Could you check a few things on this model? Use its own coordinates, in mm. A direction names the side the tool comes from. Coordinates: 2 decimals unless noted, no trailing zeros. Order: outer loops, then holes, each group sorted by start corner. A loop starts at its lowest first (then second) coordinate and runs counter-clockwise, first axis right, second up. Notation, with made-up numbers: (31.5, -22) - (62.5, -22) arc R20 cw to (62.5, 1) - close; hole circle Ø3 at (-32, -33). An arc over 180 degrees is marked (long way). Answer as CSV lines item,"result". Start each with the question number.
1. I want a section at B-B, the plane x = 13.25. List the corners of the cut face in (y, z) for me (3 decimals), and give its area (3 significant figures).
2. I want a section at A-A, the plane z = 0. List the corners of the cut face in (x, y) for me (3 decimals), and give its area (3 significant figures).
3. Thinking about a two-plate mould opening in Z: for faces 4 (the face through (8.112, -0.034, -0.774)), 5 (the face through (2.48, 2.87, 6.93)), 6 (the face through (6.88, 0.15, -3.5)), which applies, released by +Z, released by -Z, zero draft, split by the parting line, or undercut?
4. For faces 1 (the face through (7.404, -3, 5)), 2 (the face through (3.48, 0.15, -4)), 3 (the face through (13.38, -1.05, 3.34)), which set-ups out of +Z, -Z, +X, -X, +Y, -Y let a thin tool reach every point of the face, with its end or its side?
5. I want a section at D-D, the plane x = 8.5. List the corners of the cut face in (y, z) for me (3 decimals).
6. For pin 1 (1.5 mm diameter, centred on x = 4.5, z = 0, fed in from -Y); pin 2 (1 mm diameter, centred on x = 7.5, z = 1.5, fed in from -Y), each with a flat end and sliding along its axis, tell me the tip position at first contact or that it passes through.
7. I need wall thicknesses on probe 1 along X at (y, z) = (0, -1.95); probe 2 along X at (y, z) = (0, 4.5); probe 3 along Z at (x, y) = (9.25, 0) (3 decimals). Which ranges of each line are inside material? Lowest first, please.
8. I want a section at C-C, the plane y = 0. Count the separate pieces of the cut face and the enclosed holes in it, and give its area (3 significant figures).
from build123d import *

# Parameters (mm, degrees)
F2_R     = 0.5
F3_DEPTH = 12.5


with BuildPart() as f1:
    # F0 (on Front) → F1 (revolve)
    with BuildSketch(Plane.XZ):
        Polygon((1, 7.5), (0, 8.5), (0, 0.775), (16, 0.775), (16, 4), (15.404123, 3.5), (11.404123, 3.5), (11.404123, 5.5), (7.404123, 5.5), (7.404123, 6.5), (4.004123, 6.5), (4.004123, 7.5), align=None)
    revolve(axis=Axis((6.044726, 0, 0), (1, 0, 0)))

    # F2 (on Top) → F3 (cut, symmetric)
    with BuildSketch(Plane.XY):
        with Locations((3.004123, 0)):
            Circle(F2_R)
        with Locations((6.404123, 0)):
            Circle(F2_R)
        with Locations((10.404123, 0)):
            Circle(F2_R)
        with Locations((13.003722, 0)):
            Circle(F2_R)
    extrude(amount=F3_DEPTH, both=True, mode=Mode.SUBTRACT)


solid = f1.part
Solved:
1,outline,"(-0.435, -3.473) - (-0.435, -0.641) arc R0.775 cw to (-0.435, 0.641) - (-0.435, 3.473) arc R3.5 ccw to start; (0.435, -3.473) arc R3.5 ccw to (0.435, 3.473) - (0.435, 0.641) arc R0.775 cw to (0.435, -0.641) - close"
1,area,"31.8 mm2"
2,outline,"(0, -8.5) - (1, -7.5) - (4.004, -7.5) - (4.004, -6.5) - (7.404, -6.5) - (7.404, -5.5) - (11.404, -5.5) - (11.404, -3.5) - (15.404, -3.5) - (16, -4) - (16, -0.775) - (0, -0.775) - close; (0, 0.775) - (16, 0.775) - (16, 4) - (15.404, 3.5) - (11.404, 3.5) - (11.404, 5.5) - (7.404, 5.5) - (7.404, 6.5) - (4.004, 6.5) - (4.004, 7.5) - (1, 7.5) - (0, 8.5) - close"
2,area,"157 mm2"
3,face 4,"undercut"
3,face 5,"split by the parting line"
3,face 6,"zero draft"
4,face 1,"+X"
4,face 2,"+Z, -Z"
4,face 3,"none"
5,outline,"circle Ø11 at (0, 0); hole circle Ø1.55 at (0, 0)"
6,pin 1,"stops at y = -7.5"
6,pin 2,"stops at y = -6.42"
7,probe 1,"x = 0 to 2.5, 3.5 to 5.9, 6.9 to 9.9, 10.9 to 12.5, 13.5 to 16"
7,probe 2,"x = 0 to 2.5, 3.5 to 5.9, 6.9 to 9.9, 10.9 to 11.4"
7,probe 3,"z = -5.5 to -0.775, 0.775 to 5.5"
8,separate pieces,"10"
8,enclosed holes,"0"
8,area,"117 mm2"
